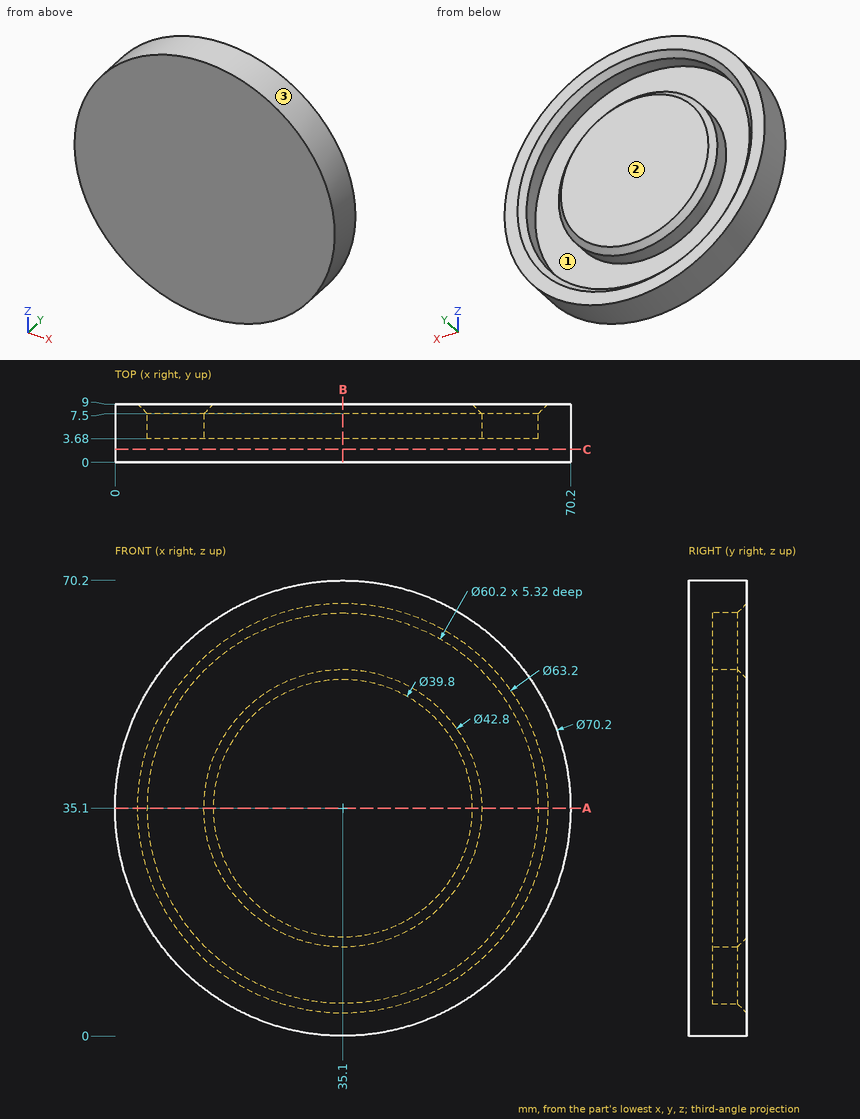
Geometry check sheet. Reference: drawing and pictorial views, mm from the part's lowest x, y, z. Round coordinates to 2 decimals unless told otherwise and drop trailing zeros. Loops run counter-clockwise (first coordinate to the right, second up) from the corner with the lowest first, then second, coordinate; pieces in that order, holes last. Notation, with made-up numbers: (-14, 16.25) - (13, 16.25) arc R34 ccw to (13, 49.25) - close; hole circle Ø3 at (66.25, -27.5). An arc over 180 degrees is marked (long way). Use a Markdown table: item, result.
Q1. Draft check along Z on the marked faces 1, 2 and 3. Enter one of: released by +Z, released by -Z, zero draft, split by the parting line, or undercut.
Solutions:
| item | result |
|---|---|
| face 1 | undercut |
| face 2 | zero draft |
| face 3 | split by the parting line |
Q2. Material ranges on line 1 (X direction, y = 6.6, z = 35.1); line 2 (X direction, y = 5, z = 19); line 3 (Z direction, x = 34, y = 7.25), recorded low to high.
Solutions:
| item | result |
|---|---|
| line 1 | x = 0 to 5, 13.7 to 56.5, 65.2 to 70.2 |
| line 2 | x = 3.91 to 9.67, 21 to 49.2, 60.53 to 66.29 |
| line 3 | z = 0.02 to 5.02, 13.73 to 56.47, 65.18 to 70.18 |
Q3. Cross-section at B-B on x = 35.1. Record the cut outline in (y, z), plus the area to 3 significant figures.
Solutions:
| item | result |
|---|---|
| outline | (0, 0) - (9, 0) - (9, 3.5) - (7.5, 5) - (3.68, 5) - (3.68, 13.7) - (7.5, 13.7) - (9, 15.2) - (9, 55) - (7.5, 56.5) - (3.68, 56.5) - (3.68, 65.2) - (7.5, 65.2) - (9, 66.7) - (9, 70.2) - (0, 70.2) - close |
| area | 535 mm2 |
Q4. Go/stop test with flat-tipped pins: P1, Ø1.5, axis at x = 11, z = 29, coming from the +Y side; P2, Ø6, axis at x = 17, z = 13.5, coming from the +Y side; P3, Ø3, axis at y = 4, z = 43.5, coming from the +X side. Record where each tip stops, or that it passes through.
Solutions:
| item | result |
|---|---|
| P1 | stops at y = 3.68 |
| P2 | stops at y = 8.58 |
| P3 | stops at x = 69.52 |
Q5. Cross-section at C-C on y = 2. Record the cut outline in (x, z).
Solutions:
| item | result |
|---|---|
| outline | circle Ø70.2 at (35.1, 35.1) |
Q6. Cross-section at A-A on z = 35.1. Record the cut outline in (x, y).
Solutions:
| item | result |
|---|---|
| outline | (0, 0) - (70.2, 0) - (70.2, 9) - (66.7, 9) - (65.2, 7.5) - (65.2, 3.68) - (56.5, 3.68) - (56.5, 7.5) - (55, 9) - (15.2, 9) - (13.7, 7.5) - (13.7, 3.68) - (5, 3.68) - (5, 7.5) - (3.5, 9) - (0, 9) - close |
